The drawing under review shows one solid part. Ordinate dimensions are in mm from its lowest x, y, z. A direction names the side the tool comes from. Round coordinates to 2 decimals unless told otherwise and drop trailing zeros. Order: outer loops, then holes, each group sorted by start corner. A loop starts at its lowest first (then second) coordinate and runs counter-clockwise, first axis right, second up. Notation, with made-up numbers: (-23.5, 56.5) -> (4.5, 56.5) arc R14 ccw to (4.5, 73.5) -> close; hole circle Ø11 at (63.5, 76). An arc over 180 degrees is marked (long way). Use a Markdown table: item, result. Add a question column.
1) Consider section B-B (z = 5.75). State the section outline as (x, y) points, plus the area to 4 significant figures.
2) Consider section D-D (x = 11). State the section outline as (y, z) points, plus the area to 4 significant figures.
3) Machinability: for the marked faces 1, 2 and 3, which of the approach directions +Z, -Z, +X, -X, +Y, -Y give a long, thin tool a straight path to every point of the face, cutting with its end or side? Answer none if there is none.
4) Consider section C-C (y = 13.5). State the section outline as (x, z) points, plus the area to 3 significant figures.
5) Clearance check with flat-ended pins moving along their axes: P1, Ø0.5, axis at x = 8.5, z = 5, coming from the +Y side; P2, Ø5, axis at y = 13.5, z = 4, coming from the +X side; P3, Ø2, axis at y = 7, z = 8, coming from the -X side; P4, Ø2, axis at y = 9.5, z = 7, coming from the -X side. State where each tip first meets the part, or that it passes through.
6) Consider section A-A (x = 6.25). State the section outline as (y, z) points, plus the area to 4 significant figures.
7) Wall thickness on line 1 along Y through (x, z) = (11, 4.5); line 2 along X through (y, z) = (8.5, 8); line 3 along Y through (x, z) = (4.5, 8.75): over which ranges is each line inside the solid? List them lowest first. Write a range as [from, to].
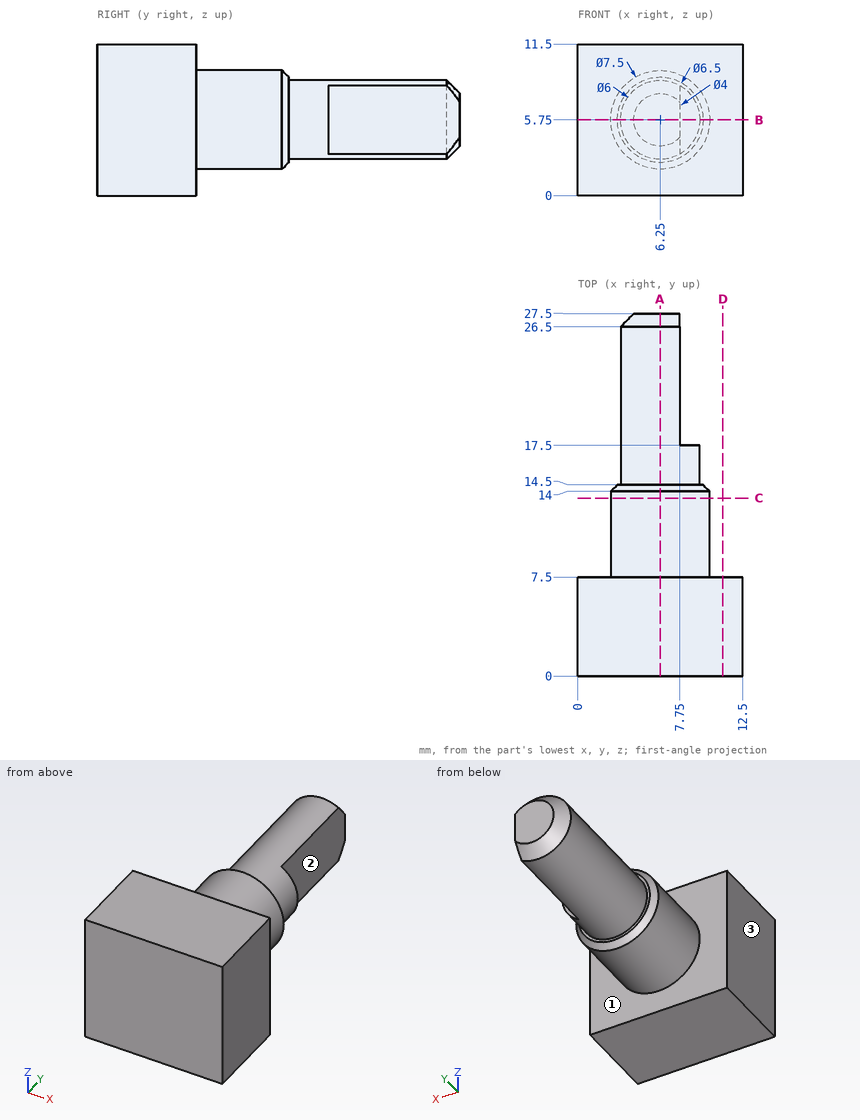
Results list:
| question | item | result |
|---|---|---|
| 1 | outline | (0, 0) -> (12.5, 0) -> (12.5, 7.5) -> (10, 7.5) -> (10, 14) -> (9.5, 14.5) -> (9.25, 14.5) -> (9.25, 17.5) -> (7.75, 17.5) -> (7.75, 27.5) -> (4.25, 27.5) -> (3.25, 26.5) -> (3.25, 14.5) -> (3, 14.5) -> (2.5, 14) -> (2.5, 7.5) -> (0, 7.5) -> close |
| 1 | area | 208.5 mm2 |
| 2 | outline | (0, 0) -> (7.5, 0) -> (7.5, 11.5) -> (0, 11.5) -> close |
| 2 | area | 86.25 mm2 |
| 3 | face 1 | +Y |
| 3 | face 2 | +Z, -Z, +X, +Y |
| 3 | face 3 | +Z, -Z, -X, +Y, -Y |
| 4 | outline | circle Ø7.5 at (6.25, 5.75) |
| 4 | area | 44.2 mm2 |
| 5 | P1 | y = 17.5 |
| 5 | P2 | x = 10 |
| 5 | P3 | x = 0 |
| 5 | P4 | x = 2.51 |
| 6 | outline | (0, 0) -> (7.5, 0) -> (7.5, 2) -> (14, 2) -> (14.5, 2.5) -> (14.5, 2.75) -> (26.5, 2.75) -> (27.5, 3.75) -> (27.5, 7.75) -> (26.5, 8.75) -> (14.5, 8.75) -> (14.5, 9) -> (14, 9.5) -> (7.5, 9.5) -> (7.5, 11.5) -> (0, 11.5) -> close |
| 6 | area | 215.5 mm2 |
| 7 | line 1 | [0, 7.5] |
| 7 | line 2 | [3.25, 9.25] |
| 7 | line 3 | [0, 14.28] |
